Autodesk Inventor part; units mm, degrees
ref_plane "bolt_to_nut_XY" through (4, 0, 0) normal (1, 0, 0) x (0, 0, -1)
ref_plane "bolt_to_nut_YZ" through (4, 0, 0) normal (0, 0, -1) x (0, 1, 0)
ref_plane "bolt_to_nut_ZX" through (4, 0, 0) normal (0, 1, 0) x (1, 0, 0)
sketch "Sketch_1" plane through (0, 0, 0) normal (0, 0, 1) x (1, 0, 0)
  line L0 (4, 0) -> (-2, 0)
  line L1 (-2, 0) -> (-2, 1.7)
  line L2 (-2, 1.7) -> (-1.8, 1.9)
  line L3 (-1.8, 1.9) -> (0, 1.9)
  line L4 (0, 1.9) -> (0, 1)
  line L5 (0, 1) -> (3.7545, 1)
  line L6 (3.7545, 1) -> (4, 0.7545)
  line L7 (4, 0.7545) -> (4, 0)
  line L8 (4, 0) -> (-2, 0)
revolve "Revolution1" add sketch "Sketch_1" angle 360 about axis through (4, 0, 0) along (1, 0, 0)
thread "Thread1"
sketch "Sketch_4_ALT_Drilling_1" plane through (0, 0, 0) normal (0, 0, 1) x (1, 0, 0)
  line L0 (-0.799, 0) -> (-2, 0)
  line L1 (-2, 0) -> (-2, 0.75)
  line L2 (-2, 0.75) -> (-1, 0.75)
  line L3 (-1, 0.75) -> (-0.799, 0)
  line L4 (-0.799, 0) -> (-2, 0)
revolve "Revolution2" cut sketch "Sketch_4_ALT_Drilling_1" angle 360 about axis through (-0.799, 0, 0) along (1, 0, 0)
sketch "Sketch_3" plane through (-2, 0, 0) normal (1, 0, 0) x (0, 0, -1)
  line L0 (-0.75, -0.433) -> (0, -0.866)
  line L1 (0, -0.866) -> (0.75, -0.433)
  line L2 (0.75, -0.433) -> (0.75, 0.433)
  line L3 (0.75, 0.433) -> (0, 0.866)
  line L4 (0, 0.866) -> (-0.75, 0.433)
  line L5 (-0.75, 0.433) -> (-0.75, -0.433)
extrude "Extrusion1" cut sketch "Sketch_3" along normal blind 1
ref_plane "bolt_to_nut_XY" through (4, 0, 0) normal (1, 0, 0) x (0, 0, -1)
ref_plane "bolt_to_nut_YZ" through (4, 0, 0) normal (0, 0, -1) x (0, 1, 0)
ref_plane "bolt_to_nut_ZX" through (4, 0, 0) normal (0, 1, 0) x (1, 0, 0)
ref_plane "screw1_XY" through (0, 0, 0) normal (1, 0, 0) x (0, 0, -1)
ref_plane "screw1_YZ" through (0, 0, 0) normal (0, 0, -1) x (0, 1, 0)
ref_plane "screw1_ZX" through (0, 0, 0) normal (0, 1, 0) x (1, 0, 0)
properties part number "CB2-4" material "鋼、炭素鋼"
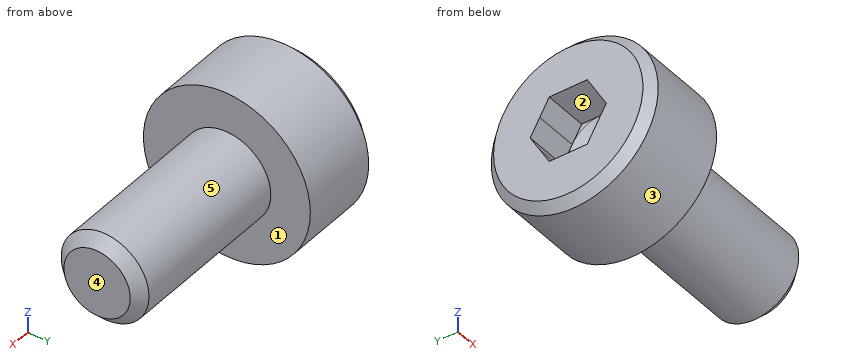
Model file for the job. Use its own axes, mm. Face numbers are marked on the shaded views. A direction names the side the tool comes from. Coordinates: 2 decimals unless noted, no trailing zeros. Write each loop counter-clockwise with the first axis right and the second up, starting at its lowest first coordinate (ties: lowest second). Pieces come first, ordered by that corner, then holes. Notation, with made-up numbers: (50, 45.25) -> (88, 45.25) arc R22 cw to (88, 65.25) -> close; hole circle Ø1 at (-32, -6). An arc over 180 degrees is marked (long way). One line per item, written item: value. Start each with the question number.
1) Pull direction Z, two halves, no side cores. Call the marked faces 1, 2 and 3: +Z half, -Z half, draft (parallel to the pull), parting line (faces both ways), or undercut.
2) Slice it at A-A on x = 1.75. Write the cut outline in (y, z), then the cut area to 3 significant figures.
3) Which spindle directions (+Z, -Z, +X, -X, +Y, -Y) get a long thin tool onto all of the face, cutting with end or side? Do the marked faces 4 and 5. Say none if no direction does.
4) Probe probe 1 along X at (y, z) = (0.7, 1); probe 2 along Y at (x, z) = (-1.5, 1.05); probe 3 along Z at (x, y) = (2.1, -0.85). List the from-to ranges inside material, lowest first.
5) Flat gauge pin, fed straight in: pin 1 Ø1.5 at (x, y) = (2, 0.5) entering from -Z. Where does the tip first touch, or does it go through?
Answers follow:
1. face 1: draft
1. face 2: undercut
1. face 3: parting line
2. outline: circle Ø2 at (0, 0)
2. area: 3.14 mm2
3. face 4: +Z, -Z, +X, +Y, -Y
3. face 5: +X
4. probe 1: -2 to 0
4. probe 2: -1.58 to 1.58
4. probe 3: -0.53 to 0.53
5. pin 1: z = -1
